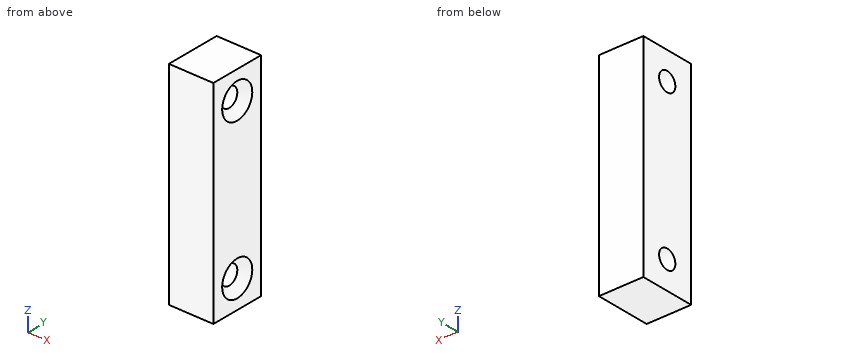
Autodesk Inventor part; units mm, degrees
ref_plane "YZ Plane" through (0, 0, 0) normal (1, 0, 0) x (0, 1, 0)
ref_plane "XZ Plane" through (0, 0, 0) normal (0, 1, 0) x (-1, 0, 0)
ref_plane "XY Plane" through (0, 0, 0) normal (0, 0, 1) x (1, 0, 0)
sketch "Sketch1" plane through (0, 0, 0) normal (0, 1, 0) x (-1, 0, 0)
  line L0 (0, 0) -> (8, 0)
  line L1 (8, 0) -> (8, -38)
  line L2 (8, -38) -> (0, -38)
  line L3 (0, -38) -> (0, 0)
  dimension "d0" = 38
  dimension "d1" = 8
extrude "Extrusion1" add sketch "Sketch1" along normal blind 10
sketch "Sketch2" plane through (0, 0, 0) normal (1, 0, 0) x (0, 0, -1)
  line L0 (0, 0) -> (0, 10)
  line L1 (38, 0) -> (38, 10)
  point P0 (5, 5)
  point P1 (33, 5)
  point P2 (38, 5)
  dimension "d4" = 5
  dimension "d5" = 5
hole "Hole1" at (0, 5, -5) at (0, 5, -33) direction (-1, 0, 0) diameter 3.4 end through all countersink diameter 6.3 countersink angle 90
properties part number "Top_End Sponge" material "Rubber, Silicone"
Input: part model. Units: mm. Frame: model coordinates. Give positions to 0.01 mm unless a question says otherwise; leave off trailing zeros. Loops run counter-clockwise (first coordinate to the right, second up) from the corner with the lowest first, then second, coordinate; pieces in that order, holes last. Notation, with made-up numbers: M 3,55.5 L 25,55.5 A20 cw 25,82.5 Z; hole C 23,51 d1. An arc over 180 degrees is marked long. Answer as CSV lines item,"result". Start each with the question number.
1. Section A-A on z = -5. Return loops of the section in (x, y).
2. Section B-B on y = 5. Return loops of the section in (x, z), plus the area to 3 significant figures.
3. Section C-C on x = -5.25. Return loops of the section in (y, z).
4. Line query: L1, parallel to Z at x = -6, y = 5; L2, parallel to Y at x = -3.25, z = -33; L3, parallel to Z at x = -2, y = 3.5. Output: solid intervals per line, ascending.
5. Pin query (flat end, axial travel): P1, Ø6, axis at y = 6, z = -11.5, coming from the +X side; P2, Ø2.5, axis at y = 5, z = -5, coming from the +X side. Return the tip coordinate at first contact, or that it passes through.
Computed values:
1,outline,"M -8,0 L 0,0 L 0,1.85 L -1.45,3.3 L -8,3.3 Z; M -8,6.7 L -1.45,6.7 L 0,8.15 L 0,10 L -8,10 Z"
2,outline,"M -8,-38 L 0,-38 L 0,-36.15 L -1.45,-34.7 L -8,-34.7 Z; M -8,-31.3 L -1.45,-31.3 L 0,-29.85 L 0,-8.15 L -1.45,-6.7 L -8,-6.7 Z; M -8,-3.3 L -1.45,-3.3 L 0,-1.85 L 0,0 L -8,0 Z"
2,area,"245 mm²"
3,outline,"M 0,-38 L 10,-38 L 10,0 L 0,0 Z; hole C 5,-33 d3.4; hole C 5,-5 d3.4"
4,L1,"z = -38 to -34.7, -31.3 to -6.7, -3.3 to 0"
4,L2,"y = 0 to 3.3, 6.7 to 10"
4,L3,"z = -38 to -33.8, -32.2 to -5.8, -4.2 to 0"
5,P1,"stops at x = 0"
5,P2,"passes through"
